from build123d import *

# Parameters (mm, degrees)
SKETCH_1_W          = 115.4
SKETCH_1_H          = 47.4
EXTRUDE_1_DEPTH     = 2
SKETCH_2_W          = 115.4
SKETCH_2_H          = 47.4
SKETCH_2_W_2        = 112.2
SKETCH_2_H_2        = 44.2
EXTRUDE_2_DEPTH     = 21
CUT_EXTRUDE_1_REACH = 67.818
SKETCH_3_W          = 87.2
SKETCH_3_H          = 29.7
SKETCH_4_W          = 10
SKETCH_4_H          = 7
CUT_EXTRUDE_2_DEPTH = 1.3
SKETCH_5_R          = 3
EXTRUDE_3_DEPTH     = 7
SKETCH_6_R          = 2
EXTRUDE_4_DEPTH     = 5
CUT_EXTRUDE_3_REACH = 65.929
SKETCH_7_R          = 1.5
SKETCH_8_R          = 4
EXTRUDE_8_DEPTH     = 3
FILLET_1_R          = 1
SKETCH_9_R          = 3
CUT_EXTRUDE_4_DEPTH = 3
CUT_EXTRUDE_5_REACH = 66.923
SKETCH_10_R         = 1.5
SKETCH_11_W         = 1.6
SKETCH_11_H         = 13
CUT_EXTRUDE_6_DEPTH = 2
FILLET_2_R          = 3.5
FILLET_3_R          = 1


# Some blends are built 0.0001 mm under size
with BuildPart() as part:
    # 草图1 → 凸台-拉伸1 (new body)
    with BuildSketch(Plane(origin=(0, 0, 0), x_dir=(1, 0, 0), z_dir=(0, 1, 0))):
        Rectangle(SKETCH_1_W, SKETCH_1_H)
    extrude(amount=EXTRUDE_1_DEPTH)

    # 草图2 → 凸台-拉伸2 (add)
    with BuildSketch(Plane(origin=(0, 2, 0), x_dir=(1, 0, 0), z_dir=(0, 1, 0))):
        Rectangle(SKETCH_2_W, SKETCH_2_H)
        Rectangle(SKETCH_2_W_2, SKETCH_2_H_2, mode=Mode.SUBTRACT)
    extrude(amount=EXTRUDE_2_DEPTH)

    # 草图3 → 切除-拉伸1 (cut, up to next)
    with BuildSketch(Plane(origin=(0, 2, 0), x_dir=(1, 0, 0), z_dir=(0, 1, 0)), mode=Mode.PRIVATE) as cut_extrude_1_sk1:
        with Locations((0, -0.75)):
            Rectangle(SKETCH_3_W, SKETCH_3_H)
    cut_extrude_1_tool1 = extrude(cut_extrude_1_sk1.sketch, amount=-CUT_EXTRUDE_1_REACH, mode=Mode.PRIVATE) & part.part
    add(cut_extrude_1_tool1.solids().sort_by_distance((0, 2, 0.75))[0], mode=Mode.SUBTRACT)

    # 草图4 → 切除-拉伸2 (cut)
    with BuildSketch(Plane(origin=(0, 2, 0), x_dir=(1, 0, 0), z_dir=(0, 1, 0))):
        with Locations((48.6, 9.6)):
            Rectangle(SKETCH_4_W, SKETCH_4_H)
    extrude(amount=-CUT_EXTRUDE_2_DEPTH, mode=Mode.SUBTRACT)

    # 草图5 → 凸台-拉伸3 (add)
    with BuildSketch(Plane(origin=(0, 2, 0), x_dir=(1, 0, 0), z_dir=(0, 1, 0))):
        with Locations(Location((50.6, -17.6, 0), (0, 0, 270))):
            Circle(SKETCH_5_R)
        with Locations(Location((50.6, 17.6, 0), (0, 0, 270))):
            Circle(SKETCH_5_R)
        with Locations(Location((-50.6, -17.6, 0), (0, 0, 270))):
            Circle(SKETCH_5_R)
        with Locations(Location((-50.6, 17.6, 0), (0, 0, 270))):
            Circle(SKETCH_5_R)
    extrude(amount=EXTRUDE_3_DEPTH)

    # 草图6 → 凸台-拉伸4 (add)
    with BuildSketch(Plane(origin=(0, 9, 0), x_dir=(1, 0, 0), z_dir=(0, 1, 0))):
        with Locations(Location((50.6, -17.6, 0), (0, 0, 270))):
            Circle(SKETCH_6_R)
        with Locations(Location((50.6, 17.6, 0), (0, 0, 270))):
            Circle(SKETCH_6_R)
        with Locations(Location((-50.6, -17.6, 0), (0, 0, 270))):
            Circle(SKETCH_6_R)
        with Locations(Location((-50.6, 17.6, 0), (0, 0, 270))):
            Circle(SKETCH_6_R)
    extrude(amount=EXTRUDE_4_DEPTH)

    # 草图7 → 切除-拉伸3 (cut, up to next)
    with BuildSketch(Plane(origin=(0, 14, 0), x_dir=(1, 0, 0), z_dir=(0, 1, 0)), mode=Mode.PRIVATE) as cut_extrude_3_sk1:
        with Locations(Location((50.6, -17.6, 0), (0, 0, 270))):
            Circle(SKETCH_7_R)
    cut_extrude_3_tool1 = extrude(cut_extrude_3_sk1.sketch, amount=-CUT_EXTRUDE_3_REACH, mode=Mode.PRIVATE) & part.part
    # 草图7 → 切除-拉伸3 (cut, up to next)
    with BuildSketch(Plane(origin=(0, 14, 0), x_dir=(1, 0, 0), z_dir=(0, 1, 0)), mode=Mode.PRIVATE) as cut_extrude_3_sk2:
        with Locations(Location((-50.6, -17.6, 0), (0, 0, 270))):
            Circle(SKETCH_7_R)
    cut_extrude_3_tool2 = extrude(cut_extrude_3_sk2.sketch, amount=-CUT_EXTRUDE_3_REACH, mode=Mode.PRIVATE) & part.part
    # 草图7 → 切除-拉伸3 (cut, up to next)
    with BuildSketch(Plane(origin=(0, 14, 0), x_dir=(1, 0, 0), z_dir=(0, 1, 0)), mode=Mode.PRIVATE) as cut_extrude_3_sk3:
        with Locations(Location((50.6, 17.6, 0), (0, 0, 270))):
            Circle(SKETCH_7_R)
    cut_extrude_3_tool3 = extrude(cut_extrude_3_sk3.sketch, amount=-CUT_EXTRUDE_3_REACH, mode=Mode.PRIVATE) & part.part
    # 草图7 → 切除-拉伸3 (cut, up to next)
    with BuildSketch(Plane(origin=(0, 14, 0), x_dir=(1, 0, 0), z_dir=(0, 1, 0)), mode=Mode.PRIVATE) as cut_extrude_3_sk4:
        with Locations(Location((-50.6, 17.6, 0), (0, 0, 270))):
            Circle(SKETCH_7_R)
    cut_extrude_3_tool4 = extrude(cut_extrude_3_sk4.sketch, amount=-CUT_EXTRUDE_3_REACH, mode=Mode.PRIVATE) & part.part
    add(cut_extrude_3_tool1.solids().sort_by_distance((50.6, 14, 17.6))[0], mode=Mode.SUBTRACT)
    add(cut_extrude_3_tool2.solids().sort_by_distance((-50.6, 14, 17.6))[0], mode=Mode.SUBTRACT)
    add(cut_extrude_3_tool3.solids().sort_by_distance((50.6, 14, -17.6))[0], mode=Mode.SUBTRACT)
    add(cut_extrude_3_tool4.solids().sort_by_distance((-50.6, 14, -17.6))[0], mode=Mode.SUBTRACT)

    # 草图8 → 凸台-拉伸8 (add)
    with BuildSketch(Plane(origin=(0, 2, 0), x_dir=(1, 0, 0), z_dir=(0, 1, 0))):
        with Locations(Location((50.6, -17.6, 0), (0, 0, 270))):
            Circle(SKETCH_8_R)
        with Locations(Location((50.6, 17.6, 0), (0, 0, 270))):
            Circle(SKETCH_8_R)
        with Locations(Location((-50.6, -17.6, 0), (0, 0, 270))):
            Circle(SKETCH_8_R)
        with Locations(Location((-50.6, 17.6, 0), (0, 0, 270))):
            Circle(SKETCH_8_R)
    extrude(amount=EXTRUDE_8_DEPTH)

    # 圆角1
    fillet_1_edges = [part.edges().sort_by_distance(p)[0] for p in [
        (50.6, 5, 14.6),
        (50.6, 5, -20.6),
        (-50.6, 5, 14.6),
        (-50.6, 5, -20.6),
    ]]
    fillet(fillet_1_edges, radius=FILLET_1_R - 0.0001)  # a hair under: the kernel refuses the full size

    # 草图9 → 切除-拉伸4 (cut)
    with BuildSketch(Plane.XZ):
        with Locations(Location((-50.6, 17.6, 0), (0, 0, 90))):
            Circle(SKETCH_9_R)
        with Locations(Location((50.6, 17.6, 0), (0, 0, 90))):
            Circle(SKETCH_9_R)
        with Locations(Location((50.6, -17.6, 0), (0, 0, 90))):
            Circle(SKETCH_9_R)
        with Locations(Location((-50.6, -17.6, 0), (0, 0, 90))):
            Circle(SKETCH_9_R)
    extrude(amount=-CUT_EXTRUDE_4_DEPTH, mode=Mode.SUBTRACT)

    # 草图10 → 切除-拉伸5 (cut, up to next)
    with BuildSketch(Plane(origin=(0, 5, 0), x_dir=(1, 0, 0), z_dir=(0, 1, 0)), mode=Mode.PRIVATE) as cut_extrude_5_sk1:
        with Locations(Location((50.6, -17.6, 0), (0, 0, 270))):
            Circle(SKETCH_10_R)
    cut_extrude_5_tool1 = extrude(cut_extrude_5_sk1.sketch, amount=-CUT_EXTRUDE_5_REACH, mode=Mode.PRIVATE) & part.part
    # 草图10 → 切除-拉伸5 (cut, up to next)
    with BuildSketch(Plane(origin=(0, 5, 0), x_dir=(1, 0, 0), z_dir=(0, 1, 0)), mode=Mode.PRIVATE) as cut_extrude_5_sk2:
        with Locations(Location((50.6, 17.6, 0), (0, 0, 270))):
            Circle(SKETCH_10_R)
    cut_extrude_5_tool2 = extrude(cut_extrude_5_sk2.sketch, amount=-CUT_EXTRUDE_5_REACH, mode=Mode.PRIVATE) & part.part
    # 草图10 → 切除-拉伸5 (cut, up to next)
    with BuildSketch(Plane(origin=(0, 5, 0), x_dir=(1, 0, 0), z_dir=(0, 1, 0)), mode=Mode.PRIVATE) as cut_extrude_5_sk3:
        with Locations(Location((-50.6, 17.6, 0), (0, 0, 270))):
            Circle(SKETCH_10_R)
    cut_extrude_5_tool3 = extrude(cut_extrude_5_sk3.sketch, amount=-CUT_EXTRUDE_5_REACH, mode=Mode.PRIVATE) & part.part
    # 草图10 → 切除-拉伸5 (cut, up to next)
    with BuildSketch(Plane(origin=(0, 5, 0), x_dir=(1, 0, 0), z_dir=(0, 1, 0)), mode=Mode.PRIVATE) as cut_extrude_5_sk4:
        with Locations(Location((-50.6, -17.6, 0), (0, 0, 270))):
            Circle(SKETCH_10_R)
    cut_extrude_5_tool4 = extrude(cut_extrude_5_sk4.sketch, amount=-CUT_EXTRUDE_5_REACH, mode=Mode.PRIVATE) & part.part
    add(cut_extrude_5_tool1.solids().sort_by_distance((50.6, 5, 17.6))[0], mode=Mode.SUBTRACT)
    add(cut_extrude_5_tool2.solids().sort_by_distance((50.6, 5, -17.6))[0], mode=Mode.SUBTRACT)
    add(cut_extrude_5_tool3.solids().sort_by_distance((-50.6, 5, -17.6))[0], mode=Mode.SUBTRACT)
    add(cut_extrude_5_tool4.solids().sort_by_distance((-50.6, 5, 17.6))[0], mode=Mode.SUBTRACT)

    # 草图11 → 切除-拉伸6 (cut)
    with BuildSketch(Plane(origin=(0, 23, 0), x_dir=(1, 0, 0), z_dir=(0, 1, 0))):
        with Locations((-56.9, -0.15)):
            Rectangle(SKETCH_11_W, SKETCH_11_H)
    extrude(amount=-CUT_EXTRUDE_6_DEPTH, mode=Mode.SUBTRACT)

    # 圆角2
    # the kernel refuses this fillet: 3.5 mm, written as the material it takes off along each edge
    with BuildSketch(Plane(origin=(66.45, 0, 23.7), x_dir=(0, 0, -1), z_dir=(-1, 0, 0)), Plane(origin=(-66.45, 0, -23.7), x_dir=(0, 0, 1), z_dir=(1, 0, 0))) as fillet_2_piece_1:
        with BuildLine():
            CenterArc((FILLET_2_R, -FILLET_2_R), FILLET_2_R, 90, 90)
            Line((0, -FILLET_2_R), (0, 0))
            Line((0, 0), (FILLET_2_R, 0))
        make_face()
    extrude(amount=132.9, mode=Mode.SUBTRACT)

    # 圆角3
    # the kernel refuses this fillet: 1 mm, written as the material it adds along each edge
    with BuildSketch(Plane(origin=(-58.6, 2, 22.1), x_dir=(0, 0, -1), z_dir=(1, 0, 0))) as fillet_3_piece_1_section:
        with BuildLine():
            CenterArc((FILLET_3_R, FILLET_3_R), FILLET_3_R, 180, 90)
            Line((0, FILLET_3_R), (0, 0))
            Line((0, 0), (FILLET_3_R, 0))
        make_face()
    fillet_3_piece_1 = extrude(amount=117.2, mode=Mode.PRIVATE)
    fillet_3_piece_1 = split(fillet_3_piece_1, bisect_by=Plane(origin=(-57.7, 2.223988989, 21.878062935), z_dir=(1, 0, 0)), keep=Keep.TOP, mode=Mode.PRIVATE)
    fillet_3_piece_1 = split(fillet_3_piece_1, bisect_by=Plane(origin=(57.7, 2.223988989, 21.878062935), z_dir=(-1, 0, 0)), keep=Keep.TOP, mode=Mode.PRIVATE)
    add(fillet_3_piece_1)
    with BuildSketch(Plane(origin=(58.6, 2, -22.1), x_dir=(0, 0, 1), z_dir=(-1, 0, 0))) as fillet_3_piece_2_section:
        with BuildLine():
            CenterArc((FILLET_3_R, FILLET_3_R), FILLET_3_R, 180, 90)
            Line((0, FILLET_3_R), (0, 0))
            Line((0, 0), (FILLET_3_R, 0))
        make_face()
    fillet_3_piece_2 = extrude(amount=117.2, mode=Mode.PRIVATE)
    fillet_3_piece_2 = split(fillet_3_piece_2, bisect_by=Plane(origin=(-57.7, 2.223988985, -21.878062921), z_dir=(1, 0, 0)), keep=Keep.TOP, mode=Mode.PRIVATE)
    fillet_3_piece_2 = split(fillet_3_piece_2, bisect_by=Plane(origin=(57.7, 2.223988985, -21.878062921), z_dir=(-1, 0, 0)), keep=Keep.TOP, mode=Mode.PRIVATE)
    add(fillet_3_piece_2)


solid = part.part
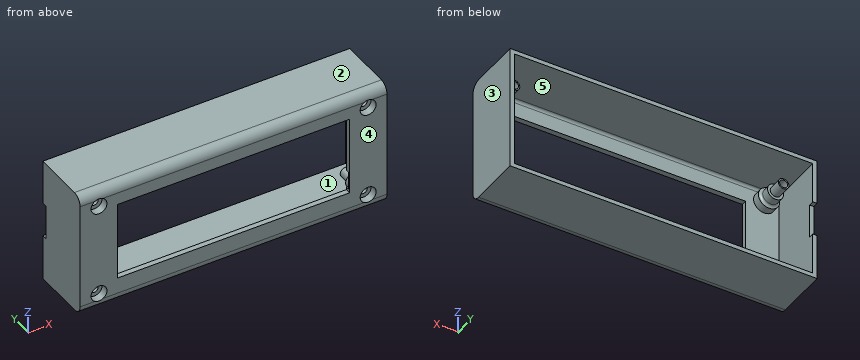
Could you check a few things on this model? Use its own coordinates, in mm. Face numbers are marked on the shaded views. A direction names the side the tool comes from. Coordinates: 2 decimals unless noted, no trailing zeros. Write each loop counter-clockwise with the first axis right and the second up, starting at its lowest first coordinate (ties: lowest second). Pieces come first, ordered by that corner, then holes. Notation, with made-up numbers: (30.5, 5.25) - (51.5, 5.25) arc R19 ccw to (51.5, 33.25) - close; hole circle Ø3 at (-30, 20.5). An arc over 180 degrees is marked (long way). Put each result on its own line as item: value. Start each with the question number.
Q1. I want a section at C-C on z = 5.5. Write out the boundary of the cut face in (x, y), plus the area to 3 significant figures.
Q2. Please list where these lines run through material, in increasing order: L1, parallel to X at y = 10.5, z = -17.6; L2, parallel to X at y = 1.8, z = 17.6; L3, parallel to X at y = 2.05, z = -17.6.
Q3. I want a section at B-B on x = 24.5. Write out the boundary of the cut face in (y, z), plus the area to 3 significant figures.
Q4. I want a section at A-A on y = 10.5. Count the separate pieces of the cut face and the enclosed holes in it, plus the area to 3 significant figures.
Q5. I'm going to push flat-ended pins straight in: P1, Ø5, axis at x = 50.5, z = -16.5, coming from the -Y side; P2, Ø1.8, axis at x = -49.5, z = 16, coming from the +Y side; P3, Ø0.5, axis at x = -56.5, z = 0, coming from the +Y side; P4, Ø1.6, axis at x = -14, y = 1.5, coming from the +Z side. Where does each tip first touch, or does it pass through?
Q6. Thinking about a two-plate mould opening in Z: for the marked faces 1, 2 and 3, which applies, pulls with the +Z half, pulls with the -Z half, needs draft (parallel to the pull), parting line crosses it, or undercut?
Q7. Which directions (+Z, -Z, +X, -X, +Y, -Y) give clear straight access to the entire face, cutting with the end or side of a thin tool? Please do the marked faces 4 and 5.
Q8. I want a section at D-D on y = 19. Write out the boundary of the cut face in (x, z).
Checks:
1. outline: (-57.7, 0) - (-43.6, 0) - (-43.6, 2) - (-56.1, 2) - (-56.1, 21) - (-57.7, 21) - close; (43.6, 0) - (57.7, 0) - (57.7, 23) - (56.1, 23) - (56.1, 2) - (43.6, 2) - close
1. area: 120 mm²
2. L1: -57.7 to -56.1, -52.6 to -52.1, -49.1 to -48.6, 48.6 to 49.1, 52.1 to 52.6, 56.1 to 57.7
2. L2: -57.7 to -53.6, -47.6 to 47.6, 53.6 to 57.7
2. L3: -57.7 to -56.1, -54.6 to -53.6, -47.6 to -46.6, 46.6 to 47.6, 53.6 to 54.6, 56.1 to 57.7
3. outline: (0, -20.2) arc R3.5 ccw to (3.5, -23.7) - (23, -23.7) - (23, -22.1) - (3, -22.1) arc R1 cw to (2, -21.1) - (2, -14.1) - (0, -14.1) - close; (0, 15.6) - (2, 15.6) - (2, 21.1) arc R1 cw to (3, 22.1) - (23, 22.1) - (23, 23.7) - (3.5, 23.7) arc R3.5 ccw to (0, 20.2) - close
3. area: 97.8 mm²
4. separate pieces: 5
4. enclosed holes: 5
4. area: 533 mm²
5. P1: y = 0
5. P2: y = 14
5. P3: y = 21
5. P4: z = 23.49
6. face 1: undercut
6. face 2: pulls with the +Z half
6. face 3: needs draft
7. face 4: +Z, -Z, +X, -X, -Y
7. face 5: +Y
8. outline: (-57.7, -23.7) - (57.7, -23.7) - (57.7, 23.7) - (-57.7, 23.7) - close; hole (-56.1, -22.1) - (56.1, -22.1) - (56.1, 22.1) - (-56.1, 22.1) - close
